Verification items for the finished model (mm, model axes). A direction names the side the tool comes from. Give positions to 0.01 mm unless a question says otherwise; leave off trailing zeros. Loops run counter-clockwise (first coordinate to the right, second up) from the corner with the lowest first, then second, coordinate; pieces in that order, holes last. Notation, with made-up numbers: (12.5, 4) -> (66.5, 4) arc R31 ccw to (66.5, 33) -> close; hole circle Ø7 at (7, 76). An arc over 180 degrees is marked (long way). Answer in a Markdown table with one row per item. Add a question column.
Q1. Section check A-A on x = 19. Enter the section's corners in (y, z).
Q2. Gauge pin test, flat ends, axial feed: P1, Ø4, axis at y = -1, z = 2.5, coming from the +X side; P2, Ø6, axis at y = 1.5, z = 1, coming from the -X side. Record the tip position at first contact, or that the pin passes through.
Q3. Section check D-D on y = -4.75. Enter the section's corners in (x, z), and give its area (3 significant figures).
Q4. Material ranges on probe 1 along Z at (x, y) = (-17.5, 0.5); probe 2 along X at (y, z) = (5.5, 2); probe 3 along X at (y, z) = (7, -2.5), recorded low to high.
Q5. Section check B-B on y = 4.5. Enter the section's corners in (x, z).
Q6. Section check C-C on z = 1. Enter the section's corners in (x, y).
Q7. Release check for a two-part mould opening along Y. For faces 3 (the face through (-20.944, 2.545, -3.134)), 4 (the face through (-18.8, -0.9, -5.5)), 5 (the face through (-1, -11.25, 0)) record: pulls with the +Y half, pulls with the -Y half, needs draft (parallel to the pull), parting line crosses it, or undercut.
Q8. Set-up check for faces 1 (the face through (-18, -10.75, 0)), 2 (the face through (19, 2, 5.25)): record each of +Z, -Z, +X, -X, +Y, -Y from which the full face is reachable in a straight line by a thin tool's end or side.
```python
from build123d import *

# Parameters (mm, degrees)
SKETCH1_W           = 42
SKETCH1_H           = 22.5
BOSS_EXTRUDE1_DEPTH = 5.75
SKETCH2_W           = 10.5
SKETCH2_H           = 21.5
CUT_EXTRUDE1_DEPTH  = 4
CUT_EXTRUDE3_DEPTH  = 12.5
SKETCH8_W           = 2.2
SKETCH8_H           = 22.5
CUT_EXTRUDE4_DEPTH  = 12.5
SKETCH3_R           = 1
BOSS_EXTRUDE2_DEPTH = 8
SKETCH4_R           = 0.5
BOSS_EXTRUDE3_DEPTH = 8
SKETCH5_R           = 1.030633651
SKETCH5_W           = 20.392034512
SKETCH5_H           = 11.098868447
CUT_EXTRUDE2_DEPTH  = 0.5


with BuildPart() as part:
    # Sketch1 → Boss-Extrude1 (new body, symmetric)
    with BuildSketch(Plane.XY):
        Rectangle(SKETCH1_W, SKETCH1_H)
    extrude(amount=BOSS_EXTRUDE1_DEPTH, both=True)

    # Sketch2 → Cut-Extrude1 (cut)
    with BuildSketch(Plane(origin=(21, 0, 0), x_dir=(0, 0, -1), z_dir=(1, 0, 0))):
        Rectangle(SKETCH2_W, SKETCH2_H)
    cut_extrude1 = extrude(amount=-CUT_EXTRUDE1_DEPTH, mode=Mode.SUBTRACT)

    # Mirror1: Cut-Extrude1 across plane
    add(cut_extrude1.mirror(Plane(origin=(0, 0, 0), x_dir=(0, 0, 1), z_dir=(1, 0, 0))), mode=Mode.SUBTRACT)

    # Sketch7 → Cut-Extrude3 (cut, through all)
    with BuildSketch(Plane.XY.offset(-5.75)):
        Polygon((24.167892902, -4.130649904), (21, -4.130649904), (17, -11.25), (17, -14.180704283), (24.167892902, -14.180704283), align=None)
    extrude(amount=CUT_EXTRUDE3_DEPTH, mode=Mode.SUBTRACT)

    # Sketch8 → Cut-Extrude4 (cut, through all)
    with BuildSketch(Plane.XY.offset(5.75)):
        with Locations((-19.9, 0)):
            Rectangle(SKETCH8_W, SKETCH8_H)
    extrude(amount=-CUT_EXTRUDE4_DEPTH, mode=Mode.SUBTRACT)

    # Sketch3 → Boss-Extrude2 (add)
    with BuildSketch(Plane(origin=(17, 0, 0), x_dir=(0, 0, -1), z_dir=(1, 0, 0))):
        with Locations((2.259944465, 7.5)):
            Circle(SKETCH3_R)
        with Locations((2.259944465, -7.5)):
            Circle(SKETCH3_R)
    extrude(amount=BOSS_EXTRUDE2_DEPTH)

    # Sketch4 → Boss-Extrude3 (add)
    with BuildSketch(Plane.ZY.offset(17)):
        with Locations((-3.364806204, 2.988148793)):
            Circle(SKETCH4_R)
        with Locations((-3.364806204, -2.988148793)):
            Circle(SKETCH4_R)
    extrude(amount=BOSS_EXTRUDE3_DEPTH)

    # Sketch5 → Cut-Extrude2 (cut)
    with BuildSketch(Plane.XY.offset(5.75)):
        with Locations((12.976825893, 7.964601522)):
            Circle(SKETCH5_R)
        with Locations((-2.003815564, 2.9231166)):
            Rectangle(SKETCH5_W, SKETCH5_H)
    extrude(amount=-CUT_EXTRUDE2_DEPTH, mode=Mode.SUBTRACT)


solid = part.part
```
Taken from the geometry:
| question | item | result |
|---|---|---|
| 1 | outline | circle Ø2 at (-7.5, -2.26); (-7.69, -5.75) -> (11.25, -5.75) -> (11.25, 5.75) -> (-7.69, 5.75) -> (-7.69, 5.25) -> (10.75, 5.25) -> (10.75, -5.25) -> (-7.69, -5.25) -> close; circle Ø2 at (7.5, -2.26) |
| 2 | P1 | stops at x = 17 |
| 2 | P2 | stops at x = -17 |
| 3 | outline | (-18.8, -5.75) -> (20.65, -5.75) -> (20.65, -5.25) -> (17, -5.25) -> (17, 5.25) -> (20.65, 5.25) -> (20.65, 5.75) -> (-18.8, 5.75) -> (-18.8, 5.25) -> (-17, 5.25) -> (-17, -5.25) -> (-18.8, -5.25) -> close |
| 3 | area | 396 mm² |
| 4 | probe 1 | z = -5.75 to -5.25, 5.25 to 5.75 |
| 4 | probe 2 | x = -17 to 17 |
| 4 | probe 3 | x = -17 to 25 |
| 5 | outline | (-18.8, -5.75) -> (21, -5.75) -> (21, -5.25) -> (17, -5.25) -> (17, 5.25) -> (21, 5.25) -> (21, 5.75) -> (8.19, 5.75) -> (8.19, 5.25) -> (-12.2, 5.25) -> (-12.2, 5.75) -> (-18.8, 5.75) -> (-18.8, 5.25) -> (-17, 5.25) -> (-17, -5.25) -> (-18.8, -5.25) -> close |
| 6 | outline | (-18.8, -11.25) -> (17, -11.25) -> (17.28, -10.75) -> (17, -10.75) -> (17, 10.75) -> (21, 10.75) -> (21, 11.25) -> (-18.8, 11.25) -> (-18.8, 10.75) -> (-17, 10.75) -> (-17, -10.75) -> (-18.8, -10.75) -> close |
| 7 | face 3 | undercut |
| 7 | face 4 | needs draft |
| 7 | face 5 | pulls with the -Y half |
| 8 | face 1 | -X |
| 8 | face 2 | +X |
